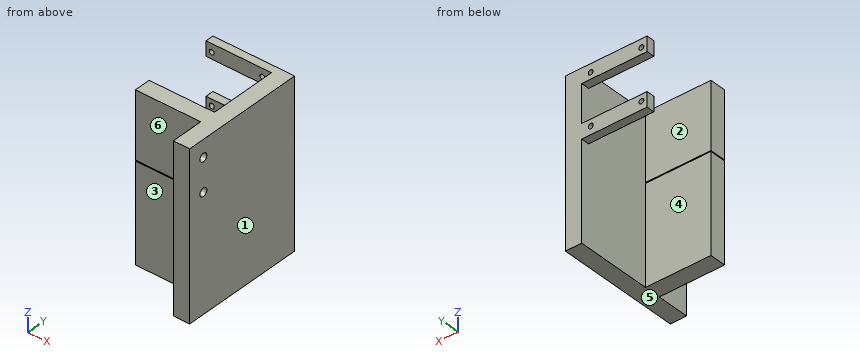
```python
from build123d import *

# Parameters (mm, degrees)
SKETCH1_W           = 41
SKETCH1_H           = 56.5
SKETCH1_H_2         = 20
SKETCH1_R           = 2.5
BOSS_EXTRUDE1_DEPTH = 10
SKETCH3_W           = 40.5
SKETCH3_H           = 10
BOSS_EXTRUDE2_DEPTH = 40
SKETCH4_W           = 9
SKETCH4_H           = 5
BOSS_EXTRUDE3_DEPTH = 40
SKETCH5_R           = 1.5
CUT_EXTRUDE1_DEPTH  = 5
SKETCH6_W           = 10
SKETCH6_H           = 76.5
SKETCH6_W_2         = 40
SKETCH6_H_2         = 10
BOSS_EXTRUDE4_DEPTH = 60


with BuildPart() as part:
    # Sketch1 → Boss-Extrude1 (new body)
    with BuildSketch(Plane(origin=(0, 0, 0), x_dir=(0, 0, -1), z_dir=(1, 0, 0))):
        with Locations((0, 28.25)):
            Rectangle(SKETCH1_W, SKETCH1_H)
        with Locations((0, -10)):
            Rectangle(SKETCH1_W, SKETCH1_H_2)
        with Locations((10, -10)):
            Circle(SKETCH1_R, mode=Mode.SUBTRACT)
        with Locations((-10, -10)):
            Circle(SKETCH1_R, mode=Mode.SUBTRACT)
    extrude(amount=BOSS_EXTRUDE1_DEPTH)

    # Sketch3 → Boss-Extrude2 (add)
    with BuildSketch(Plane.ZY):
        with Locations((0.25, 5)):
            Rectangle(SKETCH3_W, SKETCH3_H)
    extrude(amount=BOSS_EXTRUDE2_DEPTH)

    # Sketch4 → Boss-Extrude3 (add)
    with BuildSketch(Plane.ZY):
        with Locations((-16, 54)):
            Rectangle(SKETCH4_W, SKETCH4_H)
    boss_extrude3 = extrude(amount=BOSS_EXTRUDE3_DEPTH)

    # Sketch5 → Cut-Extrude1 (cut)
    with BuildSketch(Plane(origin=(0, 56.5, 0), x_dir=(1, 0, 0), z_dir=(0, 1, 0))):
        with Locations((-36.5, 15.5)):
            Circle(SKETCH5_R)
        with Locations((-5.5, 15.5)):
            Circle(SKETCH5_R)
    cut_extrude1 = extrude(amount=-CUT_EXTRUDE1_DEPTH, mode=Mode.SUBTRACT)

    # Mirror2: Boss-Extrude3, Cut-Extrude1 across plane
    add(boss_extrude3.mirror(Plane.XY))
    add(cut_extrude1.mirror(Plane.XY), mode=Mode.SUBTRACT)

    # Sketch6 → Boss-Extrude4 (add)
    with BuildSketch(Plane(origin=(0, 0, -20.5), x_dir=(-1, 0, 0), z_dir=(0, 0, -1))):
        with Locations((-5, 18.25)):
            Rectangle(SKETCH6_W, SKETCH6_H)
        with Locations((20, 5)):
            Rectangle(SKETCH6_W_2, SKETCH6_H_2)
    extrude(amount=BOSS_EXTRUDE4_DEPTH)


solid = part.part
```
Model file for the job. Use its own axes, mm. Face numbers are marked on the shaded views. A direction names the side the tool comes from. Coordinates: 2 decimals unless noted, no trailing zeros. Write each loop counter-clockwise with the first axis right and the second up, starting at its lowest first coordinate (ties: lowest second). Pieces come first, ordered by that corner, then holes. Notation, with made-up numbers: (56, -17.5) - (72, -17.5) arc R4 cw to (72, -12.5) - close; hole circle Ø9 at (-38.75, 22). An arc over 180 degrees is marked (long way). One line per item, written item: value. Start each with the question number.
1. Probe line 1 (Z direction, x = -5.5, y = 52.7); line 2 (Z direction, x = -38, y = 5.5); line 3 (X direction, y = 52, z = -15). List the from-to ranges inside material, lowest first. Write a range as from..to.
2. Slice it at C-C (y = -10). Write the cut outline in (x, z), plus the area to 3 significant figures.
3. Slice it at D-D (x = -20). Write the cut outline in (y, z).
4. Slice it at A-A (z = -15.5). Write the cut outline in (x, y), plus the area to 4 significant figures.
5. Mould opens along Y. For the marked faces 1, 2 and 3 say: released by +Y, released by -Y, zero draft, split by the parting line, or undercut.
6. Tool access for the marked faces 4, 5 and 6: list every direction of +Z, -Z, +X, -X, +Y, -Y with a clear straight run to the whole face (end or side of a thin tool).
7. Flat gauge pins, fed straight in: pin 1 (20 mm diameter, centred on x = -18.5, z = 7, fed in from -Y); pin 2 (5 mm diameter, centred on x = -36.5, z = -15.5, fed in from +Y); pin 3 (8 mm diameter, centred on y = -10, z = 10, fed in from -X); pin 4 (12 mm diameter, centred on x = -27, y = 48.5, fed in from -Z). Where does each tip first touch, or does it go through?
8. Slice it at B-B (x = -36.5). Write the cut outline in (y, z).
Answers below:
1. line 1: z = -20.5..-17, -14..-11.5, 11.5..14, 17..20.5
1. line 2: z = -80.5..-20.5, -20..20.5
1. line 3: x = -40..-37.91, -35.09..-6.91, -4.09..10
2. outline: (0, -80.5) - (10, -80.5) - (10, -12.5) - (0, -12.5) - close; (0, -7.5) - (10, -7.5) - (10, 7.5) - (0, 7.5) - close; (0, 12.5) - (10, 12.5) - (10, 20.5) - (0, 20.5) - close
2. area: 910 mm^2
3. outline: (0, -80.5) - (10, -80.5) - (10, -20.5) - (0, -20.5) - close; (0, -20) - (10, -20) - (10, 20.5) - (0, 20.5) - close; (51.5, -20.5) - (56.5, -20.5) - (56.5, -11.5) - (51.5, -11.5) - close; (51.5, 11.5) - (56.5, 11.5) - (56.5, 20.5) - (51.5, 20.5) - close
4. outline: (-40, 0) - (0, 0) - (0, -20) - (10, -20) - (10, 56.5) - (-4, 56.5) - (-4, 51.5) - (0, 51.5) - (0, 10) - (-40, 10) - close; (-40, 51.5) - (-38, 51.5) - (-38, 56.5) - (-40, 56.5) - close; (-35, 51.5) - (-7, 51.5) - (-7, 56.5) - (-35, 56.5) - close
4. area: 1,335 mm^2
5. face 1: zero draft
5. face 2: undercut
5. face 3: released by -Y
6. face 4: +Z, -Z, -X, +Y
6. face 5: -Z, +X, -X, +Y, -Y
6. face 6: +Z, -Z, -X, -Y
7. pin 1: stops at y = 0
7. pin 2: stops at y = 56.5
7. pin 3: stops at x = 0
7. pin 4: stops at z = -20.5
8. outline: (0, -80.5) - (10, -80.5) - (10, -20.5) - (0, -20.5) - close; (0, -20) - (10, -20) - (10, 20.5) - (0, 20.5) - close; (51.5, -20.5) - (56.5, -20.5) - (56.5, -17) - (51.5, -17) - close; (51.5, -14) - (56.5, -14) - (56.5, -11.5) - (51.5, -11.5) - close; (51.5, 11.5) - (56.5, 11.5) - (56.5, 14) - (51.5, 14) - close; (51.5, 17) - (56.5, 17) - (56.5, 20.5) - (51.5, 20.5) - close
